Design review of the part shown in the three views and the two pictorial views. Dimensions are in mm from the part's minimum x, y and z. Coordinates: 2 decimals unless noted, no trailing zeros. Loops run counter-clockwise (first coordinate to the right, second up) from the corner with the lowest first, then second, coordinate; pieces in that order, holes last.
Q1. Add section B-B on y = 8. Give the boundary of the cut face in (x, z).
Q2. Add section A-A on x = 39. Give the boundary of the cut face in (y, z).
Q3. Draft analysis for pull direction Y (two halves, no side actions). For the marked faces 1, 2 and 3, state which applies: released by +Y, released by -Y, zero draft, split by the parting line, or undercut.
Q4. Add section D-D on y = 5.5. Give the boundary of the cut face in (x, z).
Q5. Add section C-C on z = 2.4. Give the boundary of the cut face in (x, y).
Q6. Wall thickness on probe 1 along X at (y, z) = (8, 2); probe 2 along Y at (x, z) = (39, 1.25); probe 3 along Y at (x, z) = (48.53, 0.9): over which ranges is each line inside the solid? List them lowest first.
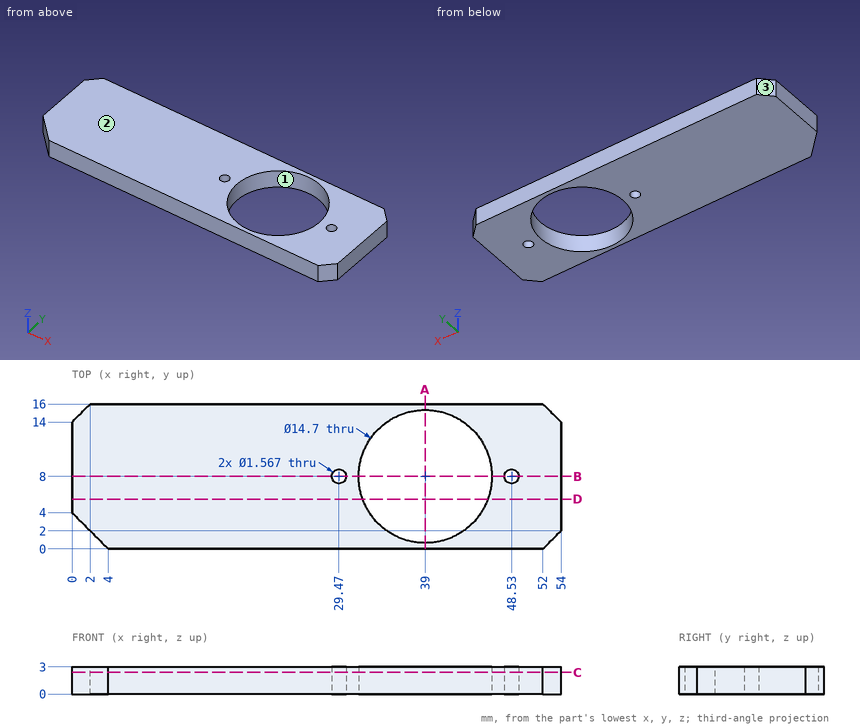
Entries:
1. outline: (0, 0) - (28.69, 0) - (28.69, 3) - (0, 3) - close; (30.25, 0) - (31.65, 0) - (31.65, 3) - (30.25, 3) - close; (46.35, 0) - (47.75, 0) - (47.75, 3) - (46.35, 3) - close; (49.31, 0) - (54, 0) - (54, 3) - (49.31, 3) - close
2. outline: (0, 0) - (0.65, 0) - (0.65, 3) - (0, 3) - close; (15.35, 0) - (16, 0) - (16, 3) - (15.35, 3) - close
3. face 1: undercut
3. face 2: zero draft
3. face 3: released by +Y
4. outline: (0, 0) - (32.09, 0) - (32.09, 3) - (0, 3) - close; (45.91, 0) - (54, 0) - (54, 3) - (45.91, 3) - close
5. outline: (0, 4) - (4, 0) - (52, 0) - (54, 2) - (54, 14) - (52, 16) - (2, 16) - (0, 14) - close; hole circle Ø1.57 at (29.47, 8); hole circle Ø14.7 at (39, 8); hole circle Ø1.57 at (48.53, 8)
6. probe 1: x = 0 to 28.69, 30.25 to 31.65, 46.35 to 47.75, 49.31 to 54
6. probe 2: y = 0 to 0.65, 15.35 to 16
6. probe 3: y = 0 to 7.22, 8.78 to 16
